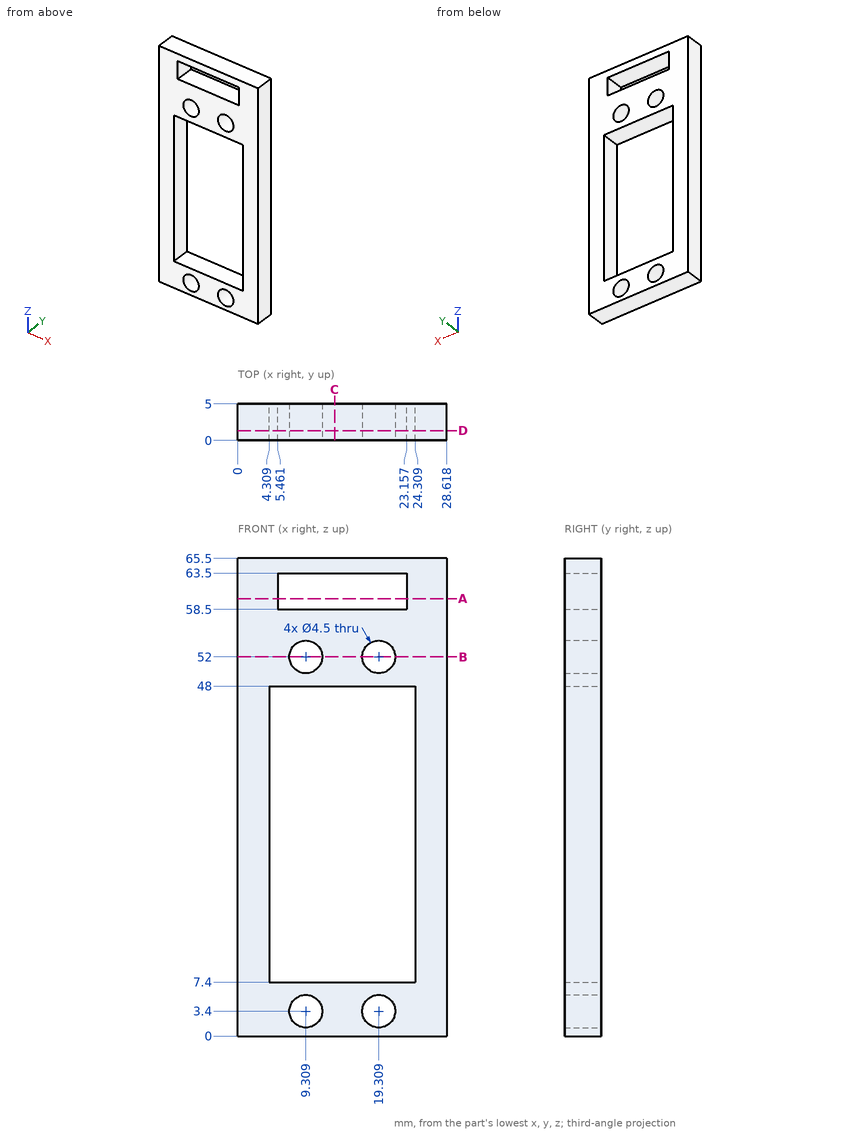
The drawing under review shows one solid part. Ordinate dimensions are in mm from its lowest x, y, z. Give positions to 0.01 mm unless a question says otherwise; leave off trailing zeros. Write each loop counter-clockwise with the first axis right and the second up, starting at its lowest first coordinate (ties: lowest second). Pieces come first, ordered by that corner, then holes. Notation, with made-up numbers: (44.25, 29) -> (64.25, 29) arc R21 ccw to (64.25, 50) -> close; hole circle Ø3 at (28.25, -12). An arc over 180 degrees is marked (long way). Use CSV: the item, a comma, the result in double quotes.
Q1. For P1, Ø2.5, axis at x = 19.31, z = 52, coming from the +Y side, flat-tipped, find the tip position at first contact; note if it passes through.
Conclusion:
P1,"through"
Q2. Take a section at B-B, the plane z = 52. Write out the cut boundary in (x, y), then the cut area to 3 significant figures.
Conclusion:
outline,"(0, 0) -> (7.06, 0) -> (7.06, 5) -> (0, 5) -> close; (11.56, 0) -> (17.06, 0) -> (17.06, 5) -> (11.56, 5) -> close; (21.56, 0) -> (28.62, 0) -> (28.62, 5) -> (21.56, 5) -> close"
area,"98.1 mm2"
Q3. To check wall thickness, follow probe 1 along X at (y, z) = (4.05, 52); probe 2 along Z at (x, y) = (7, 2.3); probe 3 along Z at (x, y) = (20, 0.95). State the ranges of each line that lie inside material, in increasing order. Write a range as [from, to].
Conclusion:
probe 1,"[0, 7.06], [11.56, 17.06], [21.56, 28.62]"
probe 2,"[0, 7.4], [48, 58.5], [63.5, 65.5]"
probe 3,"[0, 1.26], [5.54, 7.4], [48, 49.86], [54.14, 58.5], [63.5, 65.5]"
Q4. Take a section at A-A, the plane z = 60. Write out the cut boundary in (x, y), then the cut area to 3 significant figures.
Conclusion:
outline,"(0, 0) -> (5.46, 0) -> (5.46, 5) -> (0, 5) -> close; (23.16, 0) -> (28.62, 0) -> (28.62, 5) -> (23.16, 5) -> close"
area,"54.6 mm2"
Q5. Take a section at C-C, the plane x = 13.25. Write out the cut boundary in (y, z).
Conclusion:
outline,"(0, 0) -> (5, 0) -> (5, 7.4) -> (0, 7.4) -> close; (0, 48) -> (5, 48) -> (5, 58.5) -> (0, 58.5) -> close; (0, 63.5) -> (5, 63.5) -> (5, 65.5) -> (0, 65.5) -> close"
Q6. Take a section at D-D, the plane y = 1.35. Write out the cut boundary in (x, z).
Conclusion:
outline,"(0, 0) -> (28.62, 0) -> (28.62, 65.5) -> (0, 65.5) -> close; hole (4.31, 7.4) -> (24.31, 7.4) -> (24.31, 48) -> (4.31, 48) -> close; hole (5.46, 58.5) -> (23.16, 58.5) -> (23.16, 63.5) -> (5.46, 63.5) -> close; hole circle Ø4.5 at (9.31, 3.4); hole circle Ø4.5 at (9.31, 52); hole circle Ø4.5 at (19.31, 3.4); hole circle Ø4.5 at (19.31, 52)"
